The listing builds one solid part. Answer for the finished solid, in the listing's coordinates (mm). A direction names the side the tool comes from. Coordinates: 2 decimals unless noted, no trailing zeros. Write item = value, one per line. Start each with the question number.
```python
from build123d import *

# Parameters (mm, degrees)
SKETCH6_R               = 1.75
BOSS_EXTRUDE2_DEPTH     = 8
CUT_EXTRUDE4_DEPTH      = 107.173115528
CUT_EXTRUDE4_DEPTH_BACK = 107.173115528
CUT_EXTRUDE5_DEPTH      = 128.383624047
CUT_EXTRUDE5_DEPTH_BACK = 128.383624047
SKETCH8_R               = 1
SKETCH8_R_2             = 2
BOSS_EXTRUDE3_DEPTH     = 4.2
BOSS_EXTRUDE4_DEPTH     = 4.2


with BuildPart() as part:
    # Sketch6 → Boss-Extrude2 (new body)
    with BuildSketch(Plane(origin=(10.632574288, -81.095368055, -14.997352737), x_dir=(0.9917912583823046, 0.12573545426534224, 0.023252856537050268), z_dir=(-0.1278675087598277, 0.9752541956794009, 0.18035840433226386))):
        with BuildLine():
            Line((-58.720707619, -78.597122513), (-74.050825307, -74.287276551))
            Line((-74.050825307, -74.287276551), (-68.096662632, -53.10832599))
            Line((-68.096662632, -53.10832599), (-62.452093156, -54.695216936))
            add(Edge.make_bspline(
                [(-47.41282256, -71.448172315), (-46.98839964, -69.542379881), (-48.131042307, -66.495548615), (-50.899587461, -63.269699296), (-53.030599864, -61.025429488), (-55.421207388, -59.185223607), (-58.285739447, -56.985315978), (-60.74445703, -55.433736114), (-62.452093156, -54.695216936)],
                knots=[0, 0, 0, 0, 0.242004987, 0.382339127, 0.541586979, 0.632723015, 0.764707251, 1, 1, 1, 1], degree=3))
            ThreePointArc((-47.41282256, -71.448172315), (-51.536232304, -77.44357473), (-58.720707619, -78.597122513))
        make_face()
        with Locations(Location((-56.475493646, -69.630875245, 0), (0, 0, 270))):
            Circle(SKETCH6_R, mode=Mode.SUBTRACT)
    extrude(amount=BOSS_EXTRUDE2_DEPTH)

    # Sketch7 → Cut-Extrude4 (cut, two sides: drawn at the far end of the back side and taken through both)
    with BuildSketch(Plane(origin=(-24.575718662, -19.143853045, 86.09350443), x_dir=(0.9633013905822628, -0.058263627508971086, 0.26202248111903403), z_dir=(-0.2684221132885267, -0.20909392565369475, 0.9403346741200436)).offset(-CUT_EXTRUDE4_DEPTH_BACK)):
        Polygon((-40.726646112, -81.480078367), (-46.231379687, -82.217293899), (-46.664686567, -78.981823637), (-9.709847833, -74.032686551), (-9.276540953, -77.268156813), align=None)
        Polygon((-8.267725772, -84.80090478), (-39.717830931, -89.012826334), (-45.222564506, -89.750041866), (-44.789257627, -92.985512128), (-7.834418892, -88.036375042), align=None)
    extrude(amount=CUT_EXTRUDE4_DEPTH + CUT_EXTRUDE4_DEPTH_BACK, mode=Mode.SUBTRACT)

    # Sketch8 → Cut-Extrude5 (cut, two sides: drawn at the far end of the back side and taken through both)
    with BuildSketch(Plane(origin=(-48.867242553, -3.67618954, -14.766782297), x_dir=(-0.2877031657138141, -0.02164336093403552, 0.9574750405967399), z_dir=(-0.9547771830648638, -0.07182606814000152, -0.28851611156791795)).offset(-CUT_EXTRUDE5_DEPTH_BACK)):
        with Locations(Location((58.311594019, -91.780155744, 0), (0, 0, 1.243382016))):
            Circle(SKETCH8_R)
        with Locations(Location((69.605725243, -93.946396702, 0), (0, 0, 1.243382016))):
            Circle(SKETCH8_R_2)
    extrude(amount=CUT_EXTRUDE5_DEPTH + CUT_EXTRUDE5_DEPTH_BACK, mode=Mode.SUBTRACT)

    # Sketch9 → Boss-Extrude3 (add)
    with BuildSketch(Plane(origin=(9.63520772, -73.488385329, -13.590557183), x_dir=(0.9917912583823045, 0.12573545426534377, 0.023252856537050493), z_dir=(-0.12786750875982922, 0.9752541956794007, 0.18035840433226338))):
        with BuildLine():
            Line((-72.837409201, -69.971156701), (-74.050825307, -74.287276551))
            Line((-74.050825307, -74.287276551), (-67.043797112, -76.257203513))
            Line((-67.043797112, -76.257203513), (-66.509603126, -74.35707605))
            add(Edge.make_bspline(
                [(-66.509603126, -74.35707605), (-66.28129752, -73.149516128), (-68.619660453, -71.253742741), (-71.184936574, -70.487242661), (-72.837409201, -69.971156701)],
                knots=[0, 0, 0, 0, 0.375545962, 1, 1, 1, 1], degree=3))
        make_face()
    extrude(amount=BOSS_EXTRUDE3_DEPTH)

    # Sketch10 → Boss-Extrude4 (add)
    with BuildSketch(Plane(origin=(10.607000786, -80.900317216, -14.961281056), x_dir=(0.9917912583823054, 0.125735454265337, 0.023252856537049508), z_dir=(0.12786750875982242, -0.9752541956794013, -0.18035840433226552))):
        with BuildLine():
            Line((-67.043797112, 76.257203513), (-66.509603126, 74.35707605))
            add(Edge.make_bspline(
                [(-66.509603126, 74.35707605), (-66.370424117, 73.7937033), (-66.780315698, 72.705301804), (-68.402176626, 71.635929848), (-70.387506863, 70.717291368), (-72.029898632, 70.225000611), (-72.837409201, 69.971156701)],
                knots=[0, 0, 0, 0, 0.205424682, 0.379782812, 0.692407492, 1, 1, 1, 1], degree=3))
            Line((-72.837409201, 69.971156701), (-74.050825307, 74.287276551))
            Line((-74.050825307, 74.287276551), (-67.043797112, 76.257203513))
        make_face()
    extrude(amount=BOSS_EXTRUDE4_DEPTH)


solid = part.part
```
Item 1: Which of the six approach directions +Z, -Z, +X, -X, +Y, -Y give full straight-line access (tool end or side, diameter ignored) to faces 4 (the flat face through (-56.86, -93.56, 59.29)), 5 (the cylindrical face through (-49.536, -96.615, 54.059)), 6 (the flat face through (-48.76, -93.07, 50.89))?
Item 2: Each of these flat-tipped pins is pushed along its axis until it touches: pin 1 (2 mm diameter, centred on x = -59, z = 39, fed in from +Y); pin 2 (2 mm diameter, centred on y = -104, z = 48.5, fed in from +X); pin 3 (4 mm diameter, centred on x = -52, z = 42, fed in from -Y); pin 4 (1.5 mm diameter, centred on x = -61.5, y = -93.5, fed in from -Z). Where does it stop, or does it pass through?
Item 3: For a pull along Z with two mould halves and no side action, classify faces 1 (the flat face through (-60.55, -91.51, 57.39)), 2 (the cylindrical face through (-49.03, -96.09, 44.97)), 3 (the flat face through (-54.65, -95.259, 37.188)) as pulls with the +Z half, pulls with the -Z half, needs draft (parallel to the pull), parting line crosses it, or undercut.
Item 4: Consider probe 1 along Z at (x, y) = (-41.5, -95.5); probe 2 along Y at (x, z) = (-41, 57.75); probe 3 along Z at (x, y) = (-45, -98). Determine where each line is inside the solid, lowest interval first.
A:
q1.face_4 = +Z, +Y
q1.face_5 = none
q1.face_6 = +Y
q2.pin_1 = -91.99
q2.pin_2 = through
q2.pin_3 = -100.1
q2.pin_4 = 54
q3.face_1 = pulls with the +Z half
q3.face_2 = undercut
q3.face_3 = pulls with the -Z half
q4.probe_1 = 47.26 to 57.22, 58.91 to 61.22
q4.probe_2 = -101.11 to -99.27, -95.34 to -93.32
q4.probe_3 = 41.63 to 51.06, 54.28 to 54.91, 59.01 to 62.04
